Here's how the part is built. I have some questions about the finished solid (model axes, mm). Round coordinates to 2 decimals unless told otherwise and drop trailing zeros. Loops run counter-clockwise (first coordinate to the right, second up) from the corner with the lowest first, then second, coordinate; pieces in that order, holes last. Notation, with made-up numbers: M 37,-35.5 L 44,-35.5 A29 ccw 44,-6.5 Z; hole C -23.5,71 d10. An arc over 180 degrees is marked long. Answer as a JSON object with one key per item and string values.
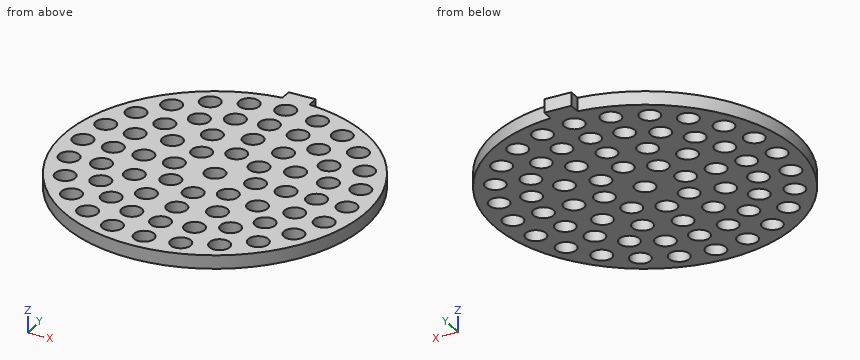
Autodesk Inventor part; units mm, degrees
ref_plane "YZ Plane" through (0, 0, 0) normal (1, 0, 0) x (0, 1, 0)
ref_plane "XZ Plane" through (0, 0, 0) normal (0, 1, 0) x (-1, 0, 0)
ref_plane "XY Plane" through (0, 0, 0) normal (0, 0, 1) x (1, 0, 0)
sketch "Эскиз1" plane through (0, 0, 0) normal (0, 0, 1) x (1, 0, 0)
  circle A0 centre (0, 0) radius 22.4
  circle A1 centre (0, 0) radius 1.5
  circle A2 centre (0, -6) radius 1.5
  circle A3 centre (0, -10.5) radius 1.5
  circle A4 centre (0, -15) radius 1.5
  circle A5 centre (0, -19.5) radius 1.5
  line L0 (-2, 21) -> (2, 21)
  line L1 (2, 21) -> (2, 24)
  line L2 (2, 24) -> (-2, 24)
  line L3 (-2, 24) -> (-2, 21)
  circle A6 centre (4.2426, -4.2426) radius 1.5
  circle A7 centre (6, 0) radius 1.5
  circle A8 centre (4.2426, 4.2426) radius 1.5
  circle A9 centre (0, 6) radius 1.5
  circle A10 centre (-4.2426, 4.2426) radius 1.5
  circle A11 centre (-6, 0) radius 1.5
  circle A12 centre (-4.2426, -4.2426) radius 1.5
  circle A13 centre (5.25, -9.0933) radius 1.5
  circle A14 centre (9.0933, -5.25) radius 1.5
  circle A15 centre (10.5, 0) radius 1.5
  circle A16 centre (9.0933, 5.25) radius 1.5
  circle A17 centre (5.25, 9.0933) radius 1.5
  circle A18 centre (0, 10.5) radius 1.5
  circle A19 centre (-5.25, 9.0933) radius 1.5
  circle A20 centre (-9.0933, 5.25) radius 1.5
  circle A21 centre (-10.5, 0) radius 1.5
  circle A22 centre (-9.0933, -5.25) radius 1.5
  circle A23 centre (-5.25, -9.0933) radius 1.5
  circle A24 centre (4.6353, -14.2658) radius 1.5
  circle A25 centre (8.8168, -12.1353) radius 1.5
  circle A26 centre (12.1353, -8.8168) radius 1.5
  circle A27 centre (14.2658, -4.6353) radius 1.5
  circle A28 centre (15, 0) radius 1.5
  circle A29 centre (14.2658, 4.6353) radius 1.5
  circle A30 centre (12.1353, 8.8168) radius 1.5
  circle A31 centre (8.8168, 12.1353) radius 1.5
  circle A32 centre (4.6353, 14.2658) radius 1.5
  circle A33 centre (0, 15) radius 1.5
  circle A34 centre (-4.6353, 14.2658) radius 1.5
  circle A35 centre (-8.8168, 12.1353) radius 1.5
  circle A36 centre (-12.1353, 8.8168) radius 1.5
  circle A37 centre (-14.2658, 4.6353) radius 1.5
  circle A38 centre (-15, 0) radius 1.5
  circle A39 centre (-14.2658, -4.6353) radius 1.5
  circle A40 centre (-12.1353, -8.8168) radius 1.5
  circle A41 centre (-8.8168, -12.1353) radius 1.5
  circle A42 centre (-4.6353, -14.2658) radius 1.5
  circle A43 centre (5.047, -18.8356) radius 1.5
  circle A44 centre (9.75, -16.8875) radius 1.5
  circle A45 centre (13.7886, -13.7886) radius 1.5
  circle A46 centre (16.8875, -9.75) radius 1.5
  circle A47 centre (18.8356, -5.047) radius 1.5
  circle A48 centre (19.5, 0) radius 1.5
  circle A49 centre (18.8356, 5.047) radius 1.5
  circle A50 centre (16.8875, 9.75) radius 1.5
  circle A51 centre (13.7886, 13.7886) radius 1.5
  circle A52 centre (9.75, 16.8875) radius 1.5
  circle A53 centre (5.047, 18.8356) radius 1.5
  circle A54 centre (0, 19.5) radius 1.5
  circle A55 centre (-5.047, 18.8356) radius 1.5
  circle A56 centre (-9.75, 16.8875) radius 1.5
  circle A57 centre (-13.7886, 13.7886) radius 1.5
  circle A58 centre (-16.8875, 9.75) radius 1.5
  circle A59 centre (-18.8356, 5.047) radius 1.5
  circle A60 centre (-19.5, 0) radius 1.5
  circle A61 centre (-18.8356, -5.047) radius 1.5
  circle A62 centre (-16.8875, -9.75) radius 1.5
  circle A63 centre (-13.7886, -13.7886) radius 1.5
  circle A64 centre (-9.75, -16.8875) radius 1.5
  circle A65 centre (-5.047, -18.8356) radius 1.5
  dimension "d1" = 3
  dimension "d2" = 3
  dimension "d3" = 3
  dimension "d4" = 3
  dimension "d5" = 3
  dimension "d6" = 4
  dimension "d7" = 3
  dimension "d10" = 360
  dimension "d14" = 360
  dimension "d18" = 360
  dimension "d22" = 360
extrude "Выдавливание1" add sketch "Эскиз1" along normal blind 2
properties part number "Матрица"
Item 1: For P1, Ø3.5, axis at x = 4.64, y = 14.27, coming from the +Z side, with a flat end and sliding along its axis, tell me the tip position at first contact or that it passes through.
Solution:
{"P1": "stops at z = 2"}
Item 2: I want a section at A-A on x = 19.5. List the corners of the cut face in (y, z) for me.
Solution:
{"outline": "M -11.02,0 L -6.39,0 L -6.39,2 L -11.02,2 Z; M -3.7,0 L -1.5,0 L -1.5,2 L -3.7,2 Z; M 1.5,0 L 3.7,0 L 3.7,2 L 1.5,2 Z; M 6.39,0 L 11.02,0 L 11.02,2 L 6.39,2 Z"}
Item 3: If I drill on L1, parallel to Y at x = 19.5, z = 1.05; L2, parallel to X at y = -3, z = 0.8; L3, parallel to X at y = -8, z = 0.7, over which ranges is the centre line in solid material (lowest first)? Write a range as from..to.
Solution:
{"L1": "y = -11.02..-6.39, -3.7..-1.5, 1.5..3.7, 6.39..11.02", "L2": "x = -22.2..-5.08, -3.4..3.4, 5.08..22.2", "L3": "x = -20.92..-13.39, -10.88..-6.28, -4.22..4.22, 6.28..10.88, 13.39..20.92"}
Item 4: I want a section at B-B on y = -9.75. Count the separate pieces of the cut face and the enclosed holes in it, plus the area to 3 significant figures.
Solution:
{"separate pieces": "8", "enclosed holes": "0", "area": "43.3 mm2"}
